For this review, take the finished solid that the model builds, in its own axes (mm). A direction names the side the tool comes from. Give positions to 0.01 mm unless a question says otherwise; leave off trailing zeros. Order: outer loops, then holes, each group sorted by start corner. A loop starts at its lowest first (then second) coordinate and runs counter-clockwise, first axis right, second up. Notation, with made-up numbers: (-18, 87.25) - (-8, 87.25) arc R17 ccw to (-8, 104.25) - close; hole circle Ø1 at (35, 27.25). An arc over 180 degrees is marked (long way). Use a Markdown table: item, result. Add a question column.
1) Machinability: for faces 4 (the face through (-42, -195, 10)), 5 (the face through (15, -14, 10)), which of the approach directions +Z, -Z, +X, -X, +Y, -Y give a long, thin tool a straight path to every point of the face, cutting with its end or side? Answer none if there is none.
2) Clearance check with flat-ended pins moving along their axes: P1, Ø5.5, axis at x = -34.036, y = -174.558, coming from the -Z side; P2, Ø3.5, axis at x = -34.036, y = -67.957, coming from the +Z side. State where each tip first meets the part, or that it passes through.
3) Wall thickness on L1, parallel to X at y = -43, z = 3.5; L2, parallel to Y at x = -29, z = 10.25 (3 decimals); L3, parallel to Y at x = -8, z = 16.75 (1 decimal): over which ranges is each line inside the solid? List them lowest first.
4) Mouldability with a two-part tool opening along Z and no side actions: class faces 1 (the face through (0.59, -375.86, 7.69)), 2 (the face through (-1, -188, 20)), 3 (the face through (-1, -421.425, 10)) as released by +Z, released by -Z, zero draft, split by the parting line, or undercut.
5) We need section C-C on z = 8.25. Give the number of separate pieces and of enclosed holes in the cut face, then the cut area to 3 significant figures.
6) We need section A-A on y = -14.5. Write out the cut boundary in (x, z), then the cut area to 3 significant figures.
7) We need section B-B on x = 25.5. Write out the cut boundary in (y, z) (3 decimals).
```python
from build123d import *

# Parameters (mm, degrees)
SKETCH1_W           = 84
SKETCH1_H           = 460
SKETCH1_R           = 6
SKETCH1_R_2         = 2
BOSS_EXTRUDE1_DEPTH = 20
SKETCH2_R           = 5
CUT_EXTRUDE1_DEPTH  = 50
SKETCH4_R           = 2.159
CUT_EXTRUDE2_DEPTH  = 20
CUT_EXTRUDE3_DEPTH  = 20
SKETCH6_R           = 2.159
CUT_EXTRUDE4_DEPTH  = 20


with BuildPart() as part:
    # Sketch1 → Boss-Extrude1 (new body)
    with BuildSketch(Plane.XY):
        with Locations((0, -191.425)):
            Rectangle(SKETCH1_W, SKETCH1_H)
        with Locations((0, -106)):
            Circle(SKETCH1_R, mode=Mode.SUBTRACT)
        with Locations((11, -106)):
            Circle(SKETCH1_R_2, mode=Mode.SUBTRACT)
        with Locations((0, -95)):
            Circle(SKETCH1_R_2, mode=Mode.SUBTRACT)
        with Locations((0, 16)):
            Circle(SKETCH1_R, mode=Mode.SUBTRACT)
        with Locations((11, 16)):
            Circle(SKETCH1_R_2, mode=Mode.SUBTRACT)
        with Locations((-11, -106)):
            Circle(SKETCH1_R_2, mode=Mode.SUBTRACT)
        with Locations((0, 27)):
            Circle(SKETCH1_R_2, mode=Mode.SUBTRACT)
        with Locations((-11, 16)):
            Circle(SKETCH1_R_2, mode=Mode.SUBTRACT)
    extrude(amount=BOSS_EXTRUDE1_DEPTH)

    # Sketch2 → Cut-Extrude1 (cut, symmetric)
    with BuildSketch(Plane(origin=(0, 0, 0), x_dir=(0, 0, -1), z_dir=(1, 0, 0))):
        with Locations((-10, -151.425)):
            Circle(SKETCH2_R)
        with Locations((-10, -371.425)):
            Circle(SKETCH2_R)
    extrude(amount=CUT_EXTRUDE1_DEPTH, both=True, mode=Mode.SUBTRACT)

    # Sketch4 → Cut-Extrude2 (cut)
    with BuildSketch(Plane.XY):
        with Locations(Location((34.036, -42.557, 0), (0, 0, 180))):
            Circle(SKETCH4_R)
        with Locations(Location((34.036, -67.957, 0), (0, 0, 180))):
            Circle(SKETCH4_R)
        with Locations(Location((-34.036, -67.957, 0), (0, 0, 180))):
            Circle(SKETCH4_R)
        with Locations(Location((-34.036, -42.557, 0), (0, 0, 180))):
            Circle(SKETCH4_R)
    extrude(amount=CUT_EXTRUDE2_DEPTH, mode=Mode.SUBTRACT)

    # Sketch5 → Cut-Extrude3 (cut)
    with BuildSketch(Plane.XY):
        with BuildLine():
            Line((15, -18.4995), (15, -9.4995))
            ThreePointArc((15, -9.4995), (14.414213562, -8.085286438), (13, -7.4995))
            Line((13, -7.4995), (-13, -7.4995))
            ThreePointArc((-13, -7.4995), (-14.414213562, -8.085286438), (-15, -9.4995))
            Line((-15, -9.4995), (-15, -18.4995))
            ThreePointArc((-15, -18.4995), (-14.414213562, -19.913713562), (-13, -20.4995))
            Line((-13, -20.4995), (13, -20.4995))
            ThreePointArc((13, -20.4995), (14.414213562, -19.913713562), (15, -18.4995))
        make_face()
    extrude(amount=CUT_EXTRUDE3_DEPTH, mode=Mode.SUBTRACT)

    # Sketch6 → Cut-Extrude4 (cut)
    with BuildSketch(Plane.XY):
        with Locations((34.036, -174.558)):
            Circle(SKETCH6_R)
        with Locations((-34.036, -174.558)):
            Circle(SKETCH6_R)
        with Locations((-34.036, -199.958)):
            Circle(SKETCH6_R)
        with Locations((34.036, -199.958)):
            Circle(SKETCH6_R)
    extrude(amount=CUT_EXTRUDE4_DEPTH, mode=Mode.SUBTRACT)


solid = part.part
```
Checked values:
| question | item | result |
|---|---|---|
| 1 | face 4 | +Z, -Z, -X, +Y, -Y |
| 1 | face 5 | +Z, -Z |
| 2 | P1 | z = 0 |
| 2 | P2 | through |
| 3 | L1 | -42 to -36.15, -31.92 to 31.92, 36.15 to 42 |
| 3 | L2 | -421.425 to -376.419, -366.431 to -156.419, -146.431 to 38.575 |
| 3 | L3 | -421.4 to -20.5, -7.5 to 38.6 |
| 4 | face 1 | undercut |
| 4 | face 2 | released by +Z |
| 4 | face 3 | zero draft |
| 5 | separate pieces | 3 |
| 5 | enclosed holes | 17 |
| 5 | area | 36,300 mm² |
| 6 | outline | (-42, 0) - (-15, 0) - (-15, 20) - (-42, 20) - close; (15, 0) - (42, 0) - (42, 20) - (15, 20) - close |
| 6 | area | 1,080 mm² |
| 7 | outline | (-421.425, 0) - (38.575, 0) - (38.575, 20) - (-421.425, 20) - close; hole circle Ø10 at (-371.425, 10); hole circle Ø10 at (-151.425, 10) |
